from build123d import *

# Parameters (mm, degrees)
BOSS_EXTRUDE1_DEPTH        = 22.225
SKETCH2_W                  = 19.812
SKETCH2_H                  = 19.558
CUT_EXTRUDE1_DEPTH         = 25.4
BOSS_EXTRUDE3_DEPTH        = 22.225
CUT_EXTRUDE2_DEPTH         = 53.968700624
BOSS_EXTRUDE4_DEPTH        = 31.115
F_6_CLEARANCE_HOLE1_REACH  = 77.492
F_6_CLEARANCE_HOLE1_BORE_R = 1.524
SKETCH13_W                 = 1.5748
SKETCH13_H                 = 1.905
BOSS_EXTRUDE5_DEPTH        = 5.08


with BuildPart() as part:
    # Sketch1 → Boss-Extrude1 (new body)
    with BuildSketch(Plane(origin=(0, 0, 0), x_dir=(1, 0, 0), z_dir=(0, 1, 0))):
        Polygon((30.08917336, 10.734503848), (40.823677208, -12.285713943), (12.7, -25.4), (0, -25.4), (0, 0), (7.068955569, 0), align=None)
    boss_extrude1 = extrude(amount=BOSS_EXTRUDE1_DEPTH)

    # Sketch2 → Cut-Extrude1 (cut)
    with BuildSketch(Plane(origin=(28.826614102, 0, -13.442070914), x_dir=(-0.4226182617407009, 0, -0.9063077870366494), z_dir=(0.9063077870366494, 0, -0.4226182617407009))):
        with Locations((-15.687469715, 9.779)):
            Rectangle(SKETCH2_W, SKETCH2_H)
    cut_extrude1 = extrude(amount=-CUT_EXTRUDE1_DEPTH, mode=Mode.SUBTRACT)

    # Mirror1: Boss-Extrude1, Cut-Extrude1 across plane
    add(boss_extrude1.mirror(Plane(origin=(0, 22.225, 0), x_dir=(0, 0, 1), z_dir=(1, 0, 0))))
    add(cut_extrude1.mirror(Plane(origin=(0, 22.225, 0), x_dir=(0, 0, 1), z_dir=(1, 0, 0))), mode=Mode.SUBTRACT)

    # Sketch4 → Boss-Extrude3 (add)
    with BuildSketch(Plane(origin=(0, 22.225, 0), x_dir=(1, 0, 0), z_dir=(0, 1, 0))):
        Polygon((22.479000043, -20.839977391), (12.7, -25.4), (22.479000043, -25.4), align=None)
    extrude(amount=-BOSS_EXTRUDE3_DEPTH)

    # Sketch6 → Cut-Extrude2 (cut, through all)
    with BuildSketch(Plane.XZ):
        with BuildLine():
            Line((19.304000043, 23.7236), (4.399409051, 23.7236))
            ThreePointArc((4.399409051, 23.7236), (3.060917478, 23.534270822), (1.827446837, 22.981138462))
            ThreePointArc((1.827446837, 22.981138462), (-1.441154453, 22.771151006), (-3.3948694, 25.4))
            Line((-3.3948694, 25.4), (19.304000043, 25.4))
            Line((19.304000043, 25.4), (19.304000043, 23.7236))
        make_face()
    cut_extrude2 = extrude(amount=-CUT_EXTRUDE2_DEPTH, mode=Mode.SUBTRACT)

    # Sketch11 → Boss-Extrude4 (add)
    with BuildSketch(Plane(origin=(0, 22.225, 0), x_dir=(1, 0, 0), z_dir=(0, 1, 0))):
        with BuildLine():
            Line((22.479000043, -25.4), (22.479000043, -20.839977391))
            Line((22.479000043, -20.839977391), (22.479000043, 0))
            Line((22.479000043, 0), (7.068955569, 0))
            Line((7.068955569, 0), (-2.920999957, 0))
            Line((-2.920999957, 0), (-2.920999957, -24.086548706))
            ThreePointArc((-2.920999957, -24.086548706), (-0.777462256, -22.542900397), (1.827446837, -22.981138462))
            ThreePointArc((1.827446837, -22.981138462), (3.060917478, -23.534270822), (4.399409051, -23.7236))
            Line((4.399409051, -23.7236), (19.304000043, -23.7236))
            Line((19.304000043, -23.7236), (19.304000043, -25.4))
            Line((19.304000043, -25.4), (22.479000043, -25.4))
        make_face()
    extrude(amount=BOSS_EXTRUDE4_DEPTH)

    # #6 Clearance Hole1 bore → #6 Clearance Hole1 (cut, up to next)
    with BuildSketch(Plane.XY.offset(23.7236), mode=Mode.PRIVATE) as f_6_clearance_hole1_sk1:
        with Locations((11.938000043, 9.652)):
            Circle(F_6_CLEARANCE_HOLE1_BORE_R)
    f_6_clearance_hole1_tool1 = extrude(f_6_clearance_hole1_sk1.sketch, amount=-F_6_CLEARANCE_HOLE1_REACH, mode=Mode.PRIVATE) & part.part
    # #6 Clearance Hole1 bore → #6 Clearance Hole1 (cut, up to next)
    with BuildSketch(Plane.XY.offset(23.7236), mode=Mode.PRIVATE) as f_6_clearance_hole1_sk2:
        with Locations((11.938000043, 46.228)):
            Circle(F_6_CLEARANCE_HOLE1_BORE_R)
    f_6_clearance_hole1_tool2 = extrude(f_6_clearance_hole1_sk2.sketch, amount=-F_6_CLEARANCE_HOLE1_REACH, mode=Mode.PRIVATE) & part.part
    add(f_6_clearance_hole1_tool1.solids().sort_by_distance((11.938, 9.652, 23.7236))[0], mode=Mode.SUBTRACT)
    add(f_6_clearance_hole1_tool2.solids().sort_by_distance((11.938, 46.228, 23.7236))[0], mode=Mode.SUBTRACT)

    # Mirror2: Cut-Extrude2 across plane
    add(cut_extrude2.mirror(Plane(origin=(0, 0, 0), x_dir=(0, 0, 1), z_dir=(1, 0, 0))), mode=Mode.SUBTRACT)

    # Sketch13 → Boss-Extrude5 (add)
    with BuildSketch(Plane(origin=(0, 53.34, 0), x_dir=(1, 0, 0), z_dir=(0, 1, 0))):
        with BuildLine():
            Line((4.399409051, -23.7236), (12.994000043, -23.7236))
            Line((12.994000043, -23.7236), (12.994000043, -22.1488))
            Line((12.994000043, -22.1488), (2.286000043, -22.1488))
            Line((2.286000043, -22.1488), (2.286000043, -19.6088))
            Line((2.286000043, -19.6088), (0.711200043, -19.6088))
            Line((0.711200043, -19.6088), (0.711200043, -22.528164802))
            ThreePointArc((0.711200043, -22.528164802), (1.289371273, -22.705248474), (1.827446837, -22.981138462))
            ThreePointArc((1.827446837, -22.981138462), (3.060917478, -23.534270822), (4.399409051, -23.7236))
        make_face()
        Polygon((15.076800043, 0), (3.494000043, 0), (3.494000043, -1.5748), (13.502000043, -1.5748), (15.076800043, -1.5748), align=None)
        with Locations((14.289400043, -2.5273)):
            Rectangle(SKETCH13_W, SKETCH13_H)
    extrude(amount=BOSS_EXTRUDE5_DEPTH)


solid = part.part
Input: part model. Units: mm. Frame: model coordinates. A direction names the side the tool comes from. Coordinates: 2 decimals unless noted, no trailing zeros. Loops run counter-clockwise (first coordinate to the right, second up) from the corner with the lowest first, then second, coordinate; pieces in that order, holes last. Notation, with made-up numbers: (-35, 70.25) - (16, 70.25) arc R22 ccw to (16, 86.25) - close; hole circle Ø7 at (-19.75, 28.5). An arc over 180 degrees is marked (long way). Answer in a Markdown table with one row per item. Add a question column.
Item 1: Line query: line 1 along Y through (x, z) = (13, 19); line 2 along X through (y, z) = (7, 13); line 3 along Y through (x, z) = (27, 2) (3 decimals). Output: solid intervals per line, ascending. Write a range as [from, to].
Item 2: Section query B-B on z = -3. Return the cut outline in (x, y) (3 decimals).
Item 3: Mould query, pull axis Z, two halves, no side actions, for faces 1 (the flat face through (8, 56, 1.575)), 2 (the flat face through (-2.921, 38, 12)), 3 (the flat face through (18.418, 10.957, -5.292)). Classes: released by +Z, released by -Z, zero draft, split by the parting line, or undercut.
Item 4: Section query D-D on z = 11. Return the cut outline in (x, y) (3 decimals), then the cut area to 3 significant figures.
Item 5: Section query A-A on y = 34. Return the cut outline in (x, z).
Item 6: Contact query for flat-ended pins moving along their axis: P1, Ø5.5, axis at x = 9, y = 56, coming from the -Z side; P2, Ø8, axis at y = 20.5, z = 11, coming from the -X side; P3, Ø0.9, axis at y = 55, z = 20.5, coming from the -X side; P4, Ø4, axis at x = 11.938, y = 9.652, coming from the +Z side. Output: stop coordinate, or through.
Item 7: Section query C-C on x = 9.5. Return the cut outline in (y, z) (3 decimals).
Item 8: Access query for faces 4 (the flat face through (12, 29, 23.724)), 5 (the cylindrical face through (-2.792, 20.37, 23.448)), 6 (the flat face through (-24, 19.558, 6)), 7 (the flat face through (8, 29, 0)). Directions: +Z, -Z, +X, -X, +Y, -Y. A direction counts if a zero-diameter tool reaches every point of the face in a straight line with its end or side. Return the directions, or none.
Recorded:
| question | item | result |
|---|---|---|
| 1 | line 1 | [0, 8.56], [10.75, 45.13], [47.32, 53.34] |
| 1 | line 2 | [-39.29, -32.68], [-13.13, 13.13], [32.68, 39.29] |
| 1 | line 3 | [19.558, 22.225] |
| 2 | outline | (-33.696, 19.558) - (-20.114, 19.558) - (-20.114, 0) - (-13.502, 0) - (-13.502, 22.225) - (-33.696, 22.225) - close; (13.502, 0) - (20.114, 0) - (20.114, 19.558) - (33.696, 19.558) - (33.696, 22.225) - (13.502, 22.225) - close |
| 3 | face 1 | undercut |
| 3 | face 2 | zero draft |
| 3 | face 3 | released by -Z |
| 4 | outline | (-40.224, 0) - (-36.97, 0) - (-36.97, 19.558) - (-12.198, 19.558) - (-12.198, 0) - (12.198, 0) - (12.198, 8.15) arc R1.524 cw (long way) to (12.198, 11.154) - (12.198, 19.558) - (36.97, 19.558) - (36.97, 0) - (40.224, 0) - (40.224, 22.225) - (22.479, 22.225) - (22.479, 53.34) - (-2.921, 53.34) - (-2.921, 22.225) - (-40.224, 22.225) - close; hole circle Ø3.048 at (11.938, 46.228) |
| 4 | area | 1,600 mm^2 |
| 5 | outline | (-2.92, 0) - (22.48, 0) - (22.48, 25.4) - (19.3, 25.4) - (19.3, 23.72) - (4.4, 23.72) arc R4.83 ccw to (1.83, 22.98) arc R3.43 cw to (-1.83, 22.98) arc R4.83 ccw to (-2.92, 23.49) - close |
| 6 | P1 | z = 0 |
| 6 | P2 | x = -40.82 |
| 6 | P3 | x = 0.71 |
| 6 | P4 | z = 23.72 |
| 7 | outline | (0, -1.134) - (22.225, -1.134) - (22.225, 0) - (58.42, 0) - (58.42, 1.575) - (53.34, 1.575) - (53.34, 22.149) - (58.42, 22.149) - (58.42, 23.724) - (0, 23.724) - (0, 5.213) - (19.558, 5.213) - (19.558, 1.949) - (0, 1.949) - close |
| 8 | face 4 | +Z, -X, +Y, -Y |
| 8 | face 5 | +Z, +Y, -Y |
| 8 | face 6 | -Y |
| 8 | face 7 | -Z, +Y |
